Check sheet for the modelled part. Datum: model origin and axes. Units: mm. Coordinates: 2 decimals unless noted, no trailing zeros. Order: outer loops, then holes, each group sorted by start corner. A loop starts at its lowest first (then second) coordinate and runs counter-clockwise, first axis right, second up.
1. Cross-section at C-C (z = 1.5). Enter the section's corners in (x, y) (3 decimals).
2. Cross-section at A-A (y = 139). Enter the section's corners in (x, z) (3 decimals), then the cut area to 3 significant figures.
3. Cross-section at B-B (x = -93.5). Enter the section's corners in (y, z) (3 decimals), then the cut area to 3 significant figures.
4. Thickness scan on line 1 (Y direction, x = 0, z = 0) (3 decimals); line 2 (Y direction, x = 34, z = 2.25); line 3 (X direction, y = 171, z = -1.25). Record the ranges inside material, lowest first.
5. Cross-section at D-D (x = 153). Enter the section's corners in (y, z) (3 decimals), then the cut area to 3 significant figures.
6. Gauge pin test, flat ends, axial feed: pin 1 Ø2 at (y, z) = (141, 0.5) entering from -X; pin 2 Ø1.5 at (y, z) = (237.5, -1) entering from +X (3 decimals); pin 3 Ø1 at (y, z) = (49, -1) entering from -X. Record the tip position at first contact, or that the pin passes through.
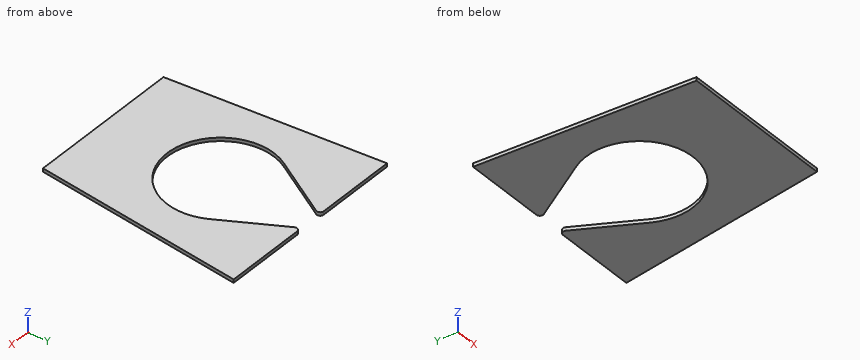
```python
from build123d import *

# Parameters (mm, degrees)
F1_DEPTH = 3.175


with BuildPart() as f1:
    # F0 (on Top) → F1 (new body, symmetric)
    with BuildSketch(Plane.XY):
        with BuildLine():
            Line((-139.7, 0), (0, 0))
            Line((0, 0), (139.7, 0))
            Line((139.7, 0), (177.8, 381))
            Line((177.8, 381), (30.934911, 381))
            ThreePointArc((30.934911, 381), (25.45374, 377.856129), (25.4, 371.537564))
            Line((25.4, 371.537564), (85.791121, 264.142763))
            ThreePointArc((85.791121, 264.142763), (95.214158, 240.834811), (98.425, 215.9))
            ThreePointArc((98.425, 215.9), (-24.934811, 120.685842), (-85.791121, 264.142763))
            Line((-85.791121, 264.142763), (-25.4, 371.537564))
            ThreePointArc((-25.4, 371.537564), (-25.45374, 377.856129), (-30.934911, 381))
            Line((-30.934911, 381), (-177.8, 381))
            Line((-177.8, 381), (-139.7, 0))
        make_face()
    extrude(amount=F1_DEPTH, both=True)


solid = f1.part
```
Data:
1. outline: (-177.8, 381) - (-139.7, 0) - (139.7, 0) - (177.8, 381) - (30.935, 381) arc R6.35 ccw to (25.4, 371.538) - (85.791, 264.143) arc R98.425 cw to (98.425, 215.9) arc R98.425 cw (long way) to (-85.791, 264.143) - (-25.4, 371.538) arc R6.35 ccw to (-30.935, 381) - close
2. outline: (-153.6, -3.175) - (-61.432, -3.175) - (-61.432, 3.175) - (-153.6, 3.175) - close; (61.432, -3.175) - (153.6, -3.175) - (153.6, 3.175) - (61.432, 3.175) - close
2. area: 1,170 mm2
3. outline: (0, -3.175) - (185.155, -3.175) - (185.155, 3.175) - (0, 3.175) - close; (246.645, -3.175) - (381, -3.175) - (381, 3.175) - (246.645, 3.175) - close
3. area: 2,030 mm2
4. line 1: y = 0 to 117.475
4. line 2: y = 0 to 123.53, 356.24 to 381
4. line 3: x = -156.8 to -87.59, 87.59 to 156.8
5. outline: (133, -3.175) - (381, -3.175) - (381, 3.175) - (133, 3.175) - close
5. area: 1,570 mm2
6. pin 1: stops at x = -153.9
6. pin 2: stops at x = 163.525
6. pin 3: stops at x = -144.65
